Part model, mm, in its own coordinate system. A direction names the side the tool comes from. Coordinates: 2 decimals unless noted, no trailing zeros. Order: outer loops, then holes, each group sorted by start corner. A loop starts at its lowest first (then second) coordinate and runs counter-clockwise, first axis right, second up.
1) Wall check: L1, parallel to Z at x = 38, y = 15.5; L2, parallel to Y at x = 24, z = 12.5; L3, parallel to Z at x = 29, y = -3. Give the ranges that are in metal, low to high.
2) Pin check, flat tips, straight feed: pin 1 Ø9 at (x, y) = (28, 17.5) entering from +Z; pin 2 Ø2 at (x, z) = (32.5, -7) entering from +Y; pin 3 Ø6 at (x, z) = (24.5, 11) entering from +Y. Stop position of each tip, or through.
3) Cut at A-A (x = 31). List the corners of the cut face in (y, z).
4) Cut at B-B (y = 8). List the corners of the cut face in (x, z), and give its area (3 significant figures).
5) Tool access for faces 1 (the flat face through (0, -11, -10)), 2 (the flat face through (20, 13, -10)): list every direction of +Z, -Z, +X, -X, +Y, -Y with a clear straight run to the whole face (end or side of a thin tool).
6) Cut at C-C (z = 5.5). List the corners of the cut face in (x, y).
```python
from build123d import *

# Parameters (mm, degrees)
F1_DEPTH = 40
F2_R     = 4


with BuildPart() as f1:
    # F0 (on Right) → F1 (new body)
    with BuildSketch(Plane.YZ):
        Polygon((-32.277047, 20), (-32.277047, -20), (27.722953, -20), (27.722953, -10), (-1.822363, -10), (-22.277047, 0), (-22.277047, 20), align=None)
    extrude(amount=F1_DEPTH)

    # F2
    f2_edges = [f1.edges().sort_by_distance(p)[0] for p in [
        (40, -27.277047, 20),
        (0, -27.277047, 20),
        (40, 27.722953, -15),
        (0, 27.722953, -15),
    ]]
    fillet(f2_edges, radius=F2_R)


solid = f1.part
```
Geometry check:
1. L1: z = -20 to -10
1. L2: y = -32.28 to -22.28
1. L3: z = -20 to -9.42
2. pin 1: stops at z = -10
2. pin 2: stops at y = -5.91
2. pin 3: stops at y = -22.28
3. outline: (-32.28, -20) - (27.72, -20) - (27.72, -10) - (-1.82, -10) - (-22.28, 0) - (-22.28, 20) - (-32.28, 20) - close
4. outline: (0, -20) - (40, -20) - (40, -10) - (0, -10) - close
4. area: 400 mm2
5. face 1: +Z, -Z, -X, +Y, -Y
5. face 2: +Z, +X, -X, +Y
6. outline: (0, -32.28) - (40, -32.28) - (40, -22.28) - (0, -22.28) - close
